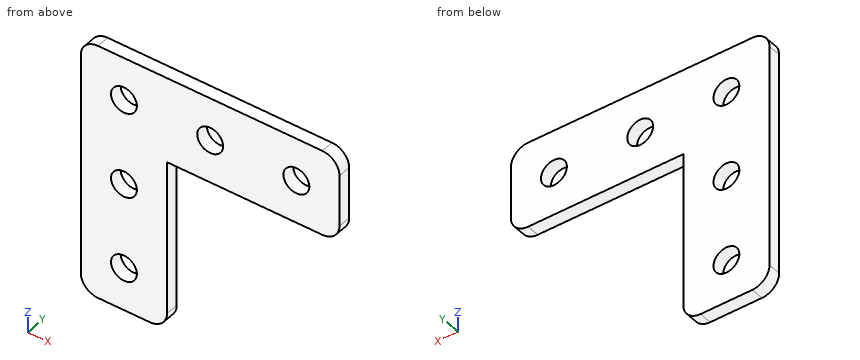
from build123d import *

# Parameters (mm, degrees)
SKETCH_2_R      = 1.5
EXTRUDE_1_DEPTH = 1.5
FILLET_1_R      = 2


with BuildPart() as part:
    # ｽｹｯﾁ2 → ﾎﾞｽ - 押し出し1 (new body)
    with BuildSketch(Plane(origin=(0, 0, 0), x_dir=(1, 0, 0), z_dir=(0, 1, 0))):
        Polygon((10, 10), (30, 10), (30, 0), (0, 0), (0, 30), (10, 30), align=None)
        with Locations(Location((5, 25, 0), (0, 0, 270))):
            Circle(SKETCH_2_R, mode=Mode.SUBTRACT)
        with Locations(Location((25, 5, 0), (0, 0, 270))):
            Circle(SKETCH_2_R, mode=Mode.SUBTRACT)
        with Locations(Location((5, 5, 0), (0, 0, 270))):
            Circle(SKETCH_2_R, mode=Mode.SUBTRACT)
        with Locations(Location((15, 5, 0), (0, 0, 270))):
            Circle(SKETCH_2_R, mode=Mode.SUBTRACT)
        with Locations(Location((5, 15, 0), (0, 0, 270))):
            Circle(SKETCH_2_R, mode=Mode.SUBTRACT)
    extrude(amount=EXTRUDE_1_DEPTH)

    # ﾌｨﾚｯﾄ1
    fillet_1_edges = [part.edges().sort_by_distance(p)[0] for p in [
        (30, 0.75, -10),
        (30, 0.75, 0),
        (0, 0.75, 0),
        (0, 0.75, -30),
        (10, 0.75, -30),
    ]]
    fillet(fillet_1_edges, radius=FILLET_1_R)


solid = part.part
The model under review builds one solid part; all positions refer to its coordinate system, in mm. Round coordinates to 2 decimals unless told otherwise and drop trailing zeros. Loops run counter-clockwise (first coordinate to the right, second up) from the corner with the lowest first, then second, coordinate; pieces in that order, holes last. Notation, with made-up numbers: (13, 29) -> (22, 29) arc R21 ccw to (22, 36) -> close; hole circle Ø5 at (71.25, 82.25). An arc over 180 degrees is marked (long way). Write item = value, one per line. Start each with the question number.
Item 1: To check wall thickness, follow L1, parallel to X at y = 0.6, z = -5; L2, parallel to X at y = 0.5, z = -25; L3, parallel to Z at x = 28, y = 0.9. State the ranges of each line that lie inside material, in increasing order.
Item 2: Take a section at A-A on z = -5. Give the boundary of the cut face in (x, y).
Item 3: Take a section at C-C on z = -25. Give the boundary of the cut face in (x, y).
Item 4: Take a section at B-B on x = 5. Give the boundary of the cut face in (y, z).
Item 5: Take a section at D-D on y = 0.4. Give the boundary of the cut face in (x, z), plus the area to 3 significant figures.
Item 6: Insertion check: pin 1 (3.5 mm diameter, centred on x = 5, z = -15, fed in from +Y); pin 2 (2.5 mm diameter, centred on x = 5, z = -5, fed in from -Y). Each pin has a flat end and moves straight along its axis. Give the tip position at first contact, or say it passes through.
Result:
q1.L1 = 0 to 3.5, 6.5 to 13.5, 16.5 to 23.5, 26.5 to 30
q1.L2 = 0 to 3.5, 6.5 to 10
q1.L3 = -10 to 0
q2.outline = (0, 0) -> (3.5, 0) -> (3.5, 1.5) -> (0, 1.5) -> close; (6.5, 0) -> (13.5, 0) -> (13.5, 1.5) -> (6.5, 1.5) -> close; (16.5, 0) -> (23.5, 0) -> (23.5, 1.5) -> (16.5, 1.5) -> close; (26.5, 0) -> (30, 0) -> (30, 1.5) -> (26.5, 1.5) -> close
q3.outline = (0, 0) -> (3.5, 0) -> (3.5, 1.5) -> (0, 1.5) -> close; (6.5, 0) -> (10, 0) -> (10, 1.5) -> (6.5, 1.5) -> close
q4.outline = (0, -30) -> (1.5, -30) -> (1.5, -26.5) -> (0, -26.5) -> close; (0, -23.5) -> (1.5, -23.5) -> (1.5, -16.5) -> (0, -16.5) -> close; (0, -13.5) -> (1.5, -13.5) -> (1.5, -6.5) -> (0, -6.5) -> close; (0, -3.5) -> (1.5, -3.5) -> (1.5, 0) -> (0, 0) -> close
q5.outline = (0, -28) arc R2 ccw to (2, -30) -> (8, -30) arc R2 ccw to (10, -28) -> (10, -10) -> (28, -10) arc R2 ccw to (30, -8) -> (30, -2) arc R2 ccw to (28, 0) -> (2, 0) arc R2 ccw to (0, -2) -> close; hole circle Ø3 at (5, -25); hole circle Ø3 at (5, -15); hole circle Ø3 at (5, -5); hole circle Ø3 at (15, -5); hole circle Ø3 at (25, -5)
q5.area = 460 mm²
q6.pin_1 = 1.5
q6.pin_2 = through
